```python
from build123d import *

# Parameters (mm, degrees)
F0_W      = 32.2
F0_H      = 54.5
F1_DEPTH  = 1.2
F3_DEPTH  = 6.7
F2_W      = 15.23
F2_H      = 15.2
F4_DEPTH  = 8.14
F2_W_2    = 6.6
F2_H_2    = 6.6
F5_DEPTH  = 6
F6_R      = 2
F7_DEPTH  = 2.5
F9_DEPTH  = 10.2
F10_DEPTH = 2
F11_DEPTH = 6
F13_DEPTH = 1.5


with BuildPart() as f1:
    # F0 (on Top) → F1 (new body)
    with BuildSketch(Plane.XY):
        Rectangle(F0_W, F0_H)
    extrude(amount=F1_DEPTH)

    # F2 (on face) → F3 (join)
    with BuildSketch(Plane.XY.offset(1.2)):
        Polygon((-7.615, -12.05), (7.615, -12.05), (16.1, -12.05), (16.1, 27.25), (-16.1, 27.25), (-16.1, -12.05), align=None)
    extrude(amount=F3_DEPTH)

    # F2 (on face) → F4 (join)
    with BuildSketch(Plane.XY.offset(1.2)):
        with Locations((0, -19.65)):
            Rectangle(F2_W, F2_H)
    extrude(amount=F4_DEPTH)

    # F2 (on face) → F5 (join)
    with BuildSketch(Plane.XY.offset(1.2)):
        with Locations((-11.8228513747, -22.7176826447)):
            Rectangle(F2_W_2, F2_H_2)
        with Locations((11.9689786807, -22.7176826447)):
            Rectangle(F2_W_2, F2_H_2)
    extrude(amount=F5_DEPTH)

    # F6 (on face) → F7 (join)
    with BuildSketch(Plane(origin=(0, 0, 0), x_dir=(1, 0, 0), z_dir=(0, 0, -1))):
        with Locations((-11.8832346052, 16.5988039225)):
            Circle(F6_R)
    extrude(amount=F7_DEPTH)

    # F8 (on face) → F9 (join)
    with BuildSketch(Plane(origin=(0, 27.25, 0), x_dir=(-1, 0, 0), z_dir=(0, 1, 0))):
        with BuildLine():
            ThreePointArc((13.5, 2.4), (9.0719637109, 5.2011282753), (8.437858313, 0))
            Line((8.437858313, 0), (12.362141687, 0))
            ThreePointArc((12.362141687, 0), (13.2011282753, 1.0719637109), (13.5, 2.4))
        make_face()
        with BuildLine():
            Line((12.362141687, 0), (8.437858313, 0))
            ThreePointArc((8.437858313, 0), (10.4, -0.7), (12.362141687, 0))
        make_face()
    extrude(amount=F9_DEPTH)

    # F8 (on face) → F10 (join)
    with BuildSketch(Plane(origin=(0, 27.25, 0), x_dir=(-1, 0, 0), z_dir=(0, 1, 0))):
        with BuildLine():
            Line((8.437858313, 0), (7, 0))
            Line((7, 0), (7, -1))
            Line((7, -1), (13.8, -1))
            Line((13.8, -1), (13.8, 0))
            Line((13.8, 0), (12.362141687, 0))
            ThreePointArc((12.362141687, 0), (10.4, -0.7), (8.437858313, 0))
        make_face()
        with BuildLine():
            Line((13.8, 5.8), (7, 5.8))
            Line((7, 5.8), (7, 0))
            Line((7, 0), (8.437858313, 0))
            ThreePointArc((8.437858313, 0), (9.0719637109, 5.2011282753), (13.5, 2.4))
            ThreePointArc((13.5, 2.4), (13.2011282753, 1.0719637109), (12.362141687, 0))
            Line((12.362141687, 0), (13.8, 0))
            Line((13.8, 0), (13.8, 5.8))
        make_face()
    extrude(amount=F10_DEPTH)

    # F8 (on face) → F11 (join)
    with BuildSketch(Plane(origin=(0, 27.25, 0), x_dir=(-1, 0, 0), z_dir=(0, 1, 0))):
        with BuildLine():
            Line((8.437858313, 0), (7, 0))
            Line((7, 0), (7, -1))
            Line((7, -1), (13.8, -1))
            Line((13.8, -1), (13.8, 0))
            Line((13.8, 0), (12.362141687, 0))
            ThreePointArc((12.362141687, 0), (10.4, -0.7), (8.437858313, 0))
        make_face()
        with BuildLine():
            Line((12.362141687, 0), (8.437858313, 0))
            ThreePointArc((8.437858313, 0), (10.4, -0.7), (12.362141687, 0))
        make_face()
    extrude(amount=-F11_DEPTH)

    # F12 (on face) → F13 (cut)
    with BuildSketch(Plane.XY.offset(9.34)):
        Polygon((-7.615, -27.25), (-3.8, -27.25), (-3.8, -23.55), (3.8, -23.55), (3.8, -27.25), (7.615, -27.25), (7.615, -12.05), (-7.615, -12.05), align=None)
    extrude(amount=-F13_DEPTH, mode=Mode.SUBTRACT)


solid = f1.part
```
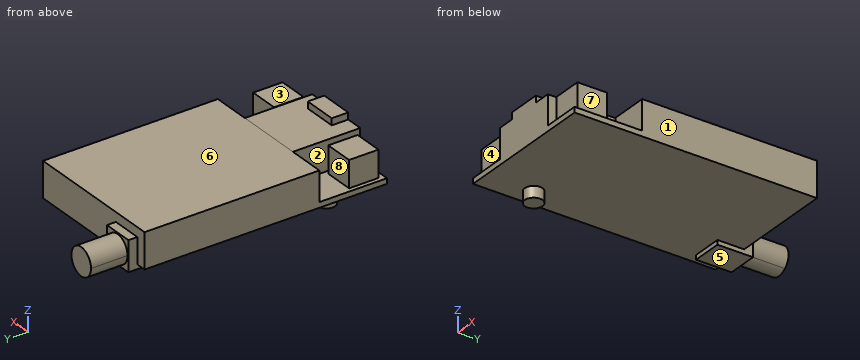
The model under review builds one solid part; all positions refer to its coordinate system, in mm. Face numbers are marked on the shaded views. A direction names the side the tool comes from. Coordinates: 2 decimals unless noted, no trailing zeros. Write each loop counter-clockwise with the first axis right and the second up, starting at its lowest first coordinate (ties: lowest second). Pieces come first, ordered by that corner, then holes.
1) We need section A-A on y = -13.5. State the section outline as (x, z) points (3 decimals), then the cut area to 3 significant figures.
2) To check wall thickness, follow probe 1 along X at (y, z) = (-20, 2.5) (3 decimals); probe 2 along Y at (x, z) = (13, 5.5); probe 3 along Y at (x, z) = (-10, 4.25). State the ranges of each line that lie inside material, in increasing order.
3) Clearance check with flat-ended pins moving along their axes: pin 1 Ø1.8 at (y, z) = (-23, 5.5) entering from +X; pin 2 Ø2 at (x, y) = (13.5, -24) entering from +Z; pin 3 Ø5 at (x, z) = (12, 4) entering from -Y. State where each tip first meets the part, or that it passes through.
4) We need section C-C on y = -2. State the section outline as (x, z) points, then the cut area to 3 significant figures.
5) Machinability: for the marked faces 4, 5, 6, 7 and 8, which of the approach directions +Z, -Z, +X, -X, +Y, -Y give a long, thin tool a straight path to every point of the face, cutting with its end or side? Answer none if there is none.
6) The part is to be moulded in two halves that separate along X. For the marked faces 1, 2 and 3, say which applies: pulls with the +X half, pulls with the -X half, needs draft (parallel to the pull), parting line crosses it, or undercut.
7) We need section B-B on x = 13. State the section outline as (y, z) points.
Answer list:
1. outline: (-16.1, 0) - (16.1, 0) - (16.1, 1.2) - (7.615, 1.2) - (7.615, 7.84) - (-7.615, 7.84) - (-7.615, 1.2) - (-16.1, 1.2) - close
1. area: 140 mm2
2. probe 1: x = -15.123 to -8.523, -7.615 to 7.615, 8.669 to 15.269
2. probe 2: y = -26.02 to -19.42, -12.05 to 27.25
2. probe 3: y = -26.02 to -19.42, -12.05 to 37.45
3. pin 1: stops at x = 15.27
3. pin 2: stops at z = 7.2
3. pin 3: stops at y = -26.02
4. outline: (-16.1, 0) - (16.1, 0) - (16.1, 7.9) - (-16.1, 7.9) - close
4. area: 254 mm2
5. face 4: +Z, -X, -Y
5. face 5: -Z, +X, -X, +Y
5. face 6: +Z, +X, -X, +Y
5. face 7: +Z, +X, -Y
5. face 8: +Z, -X
6. face 1: pulls with the +X half
6. face 2: undercut
6. face 3: needs draft
7. outline: (-27.25, 0) - (27.25, 0) - (27.25, 7.9) - (-12.05, 7.9) - (-12.05, 1.2) - (-19.42, 1.2) - (-19.42, 7.2) - (-26.02, 7.2) - (-26.02, 1.2) - (-27.25, 1.2) - close
